from build123d import *

# Parameters (mm, degrees)
SKETCH1_W           = 50
SKETCH1_H           = 50
BOSS_EXTRUDE1_DEPTH = 30
SKETCH2_R           = 2.5
CUT_EXTRUDE1_DEPTH  = 15
CUT_EXTRUDE2_REACH  = 65.443
SKETCH4_R           = 6
SKETCH5_R           = 1.5
CUT_EXTRUDE3_DEPTH  = 10
CUT_EXTRUDE4_START  = -10
SKETCH6_R           = 1.5
CUT_EXTRUDE4_DEPTH  = 10
FILLET1_R           = 4
SKETCH8_R           = 2.5
CUT_EXTRUDE5_DEPTH  = 15


with BuildPart() as part:
    # Sketch1 → Boss-Extrude1 (new body)
    with BuildSketch(Plane(origin=(0, 0, 0), x_dir=(1, 0, 0), z_dir=(0, 1, 0))):
        Rectangle(SKETCH1_W, SKETCH1_H)
    extrude(amount=BOSS_EXTRUDE1_DEPTH)

    # Sketch2 → Cut-Extrude1 (cut)
    with BuildSketch(Plane.XZ):
        with Locations(Location((0, 10, 0), (0, 0, 270))):
            Circle(SKETCH2_R)
        with Locations(Location((0, -10, 0), (0, 0, 270))):
            Circle(SKETCH2_R)
        with Locations(Location((10, 0, 0), (0, 0, 270))):
            Circle(SKETCH2_R)
        with Locations(Location((-10, 0, 0), (0, 0, 270))):
            Circle(SKETCH2_R)
        with Locations(Location((0, 0, 0), (0, 0, 270))):
            Circle(SKETCH2_R)
    extrude(amount=-CUT_EXTRUDE1_DEPTH, mode=Mode.SUBTRACT)

    # Sketch4 → Cut-Extrude2 (cut, up to next)
    with BuildSketch(Plane.ZY.offset(25), mode=Mode.PRIVATE) as cut_extrude2_sk1:
        with Locations((0, 16)):
            Circle(SKETCH4_R)
    cut_extrude2_tool1 = extrude(cut_extrude2_sk1.sketch, amount=-CUT_EXTRUDE2_REACH, mode=Mode.PRIVATE) & part.part
    add(cut_extrude2_tool1.solids().sort_by_distance((-25, 16, 0))[0], mode=Mode.SUBTRACT)

    # Sketch5 → Cut-Extrude3 (cut)
    with BuildSketch(Plane.ZY.offset(25)):
        with Locations((-8, 16)):
            Circle(SKETCH5_R)
        with Locations((8, 16)):
            Circle(SKETCH5_R)
        with Locations((0, 8)):
            Circle(SKETCH5_R)
        with Locations((0, 24)):
            Circle(SKETCH5_R)
    extrude(amount=-CUT_EXTRUDE3_DEPTH, mode=Mode.SUBTRACT)

    # Sketch6 → Cut-Extrude4 (cut)
    with BuildSketch(Plane(origin=(25, 0, 0), x_dir=(0, 0, -1), z_dir=(1, 0, 0)).offset(CUT_EXTRUDE4_START)):
        with Locations(Location((-8, 16, 0), (0, 0, 180))):
            Circle(SKETCH6_R)
        with Locations(Location((8, 16, 0), (0, 0, 180))):
            Circle(SKETCH6_R)
        with Locations(Location((0, 24, 0), (0, 0, 180))):
            Circle(SKETCH6_R)
        with Locations(Location((0, 8, 0), (0, 0, 180))):
            Circle(SKETCH6_R)
    extrude(amount=CUT_EXTRUDE4_DEPTH, mode=Mode.SUBTRACT)

    # Fillet1
    fillet1_edges = [part.edges().sort_by_distance(p)[0] for p in [
        (25, 15, 25),
        (-25, 15, 25),
        (-25, 15, -25),
        (25, 15, -25),
    ]]
    fillet(fillet1_edges, radius=FILLET1_R)

    # Sketch8 → Cut-Extrude5 (cut)
    with BuildSketch(Plane(origin=(0, 30, 0), x_dir=(1, 0, 0), z_dir=(0, 1, 0))):
        with Locations(Location((-16, 16, 0), (0, 0, 270))):
            Circle(SKETCH8_R)
        with Locations(Location((16, 16, 0), (0, 0, 270))):
            Circle(SKETCH8_R)
        with Locations(Location((16, -16, 0), (0, 0, 270))):
            Circle(SKETCH8_R)
        with Locations(Location((-16, -16, 0), (0, 0, 270))):
            Circle(SKETCH8_R)
    extrude(amount=-CUT_EXTRUDE5_DEPTH, mode=Mode.SUBTRACT)


solid = part.part
Can you work these out from the model? Positions are in its coordinate system, mm. A direction names the side the tool comes from. Coordinates: 2 decimals unless noted, no trailing zeros. Order: outer loops, then holes, each group sorted by start corner. A loop starts at its lowest first (then second) coordinate and runs counter-clockwise, first axis right, second up. Notation, with made-up numbers: (-32, 66) -> (-22, 66) arc R28 cw to (-22, 87) -> close; hole circle Ø6 at (-19.5, 49). An arc over 180 degrees is marked (long way). Use one line per item in the form item = value.
Q1. We'd pull the mould along Z, two halves only. Please class faces 6 (the face through (0, 30, 0)), 7 (the face through (-23.859, 15.21, 23.797)), 8 (the face through (-17.5, 22.6, 14)): released by +Z, released by -Z, zero draft, split by the parting line, or undercut.
From the geometry:
face_6 = zero draft
face_7 = released by +Z
face_8 = undercut
Q2. Will these pins go through, and if not, where does the flat tip stop? P1, Ø1.5, axis at y = 16.5, z = 8, coming from the +X side; P2, Ø2.5, axis at y = 8, z = 0, coming from the -X side.
From the geometry:
P1 = 15
P2 = -15
Q3. Imagine slicing it at D-D, the plane x = 5.5. List the corners of the cut face in (y, z) for me.
From the geometry:
outline = (0, -25) -> (30, -25) -> (30, 25) -> (0, 25) -> close; hole circle Ø12 at (16, 0)
Q4. Imagine slicing it at B-B, the plane y = 13. List the corners of the cut face in (x, z) for me.
From the geometry:
outline = (-25, -21) arc R4 ccw to (-21, -25) -> (21, -25) arc R4 ccw to (25, -21) -> (25, -5.2) -> (-25, -5.2) -> close; (-25, 5.2) -> (25, 5.2) -> (25, 21) arc R4 ccw to (21, 25) -> (-21, 25) arc R4 ccw to (-25, 21) -> close; hole circle Ø5 at (0, -10); hole circle Ø5 at (0, 10)
Q5. I need wall thicknesses on L1, parallel to X at y = 22.5, z = 16; L2, parallel to Z at x = 20, y = 8; L3, parallel to X at y = 18, z = -14. Which ranges of each line are inside material? Lowest first, please.
From the geometry:
L1 = -25 to -18.5, -13.5 to 13.5, 18.5 to 25
L2 = -25 to -1.5, 1.5 to 25
L3 = -25 to -17.5, -14.5 to 14.5, 17.5 to 25
Q6. Imagine slicing it at A-A, the plane x = 16. List the corners of the cut face in (y, z) for me, then the cut area to 3 significant figures.
From the geometry:
outline = (0, -25) -> (30, -25) -> (30, -18.5) -> (15, -18.5) -> (15, -13.5) -> (30, -13.5) -> (30, 13.5) -> (15, 13.5) -> (15, 18.5) -> (30, 18.5) -> (30, 25) -> (0, 25) -> close; hole circle Ø3 at (8, 0); hole circle Ø12 at (16, 0); hole circle Ø3 at (16, -8); hole circle Ø3 at (16, 8); hole circle Ø3 at (24, 0)
area = 1,210 mm²
Q7. Which directions (+Z, -Z, +X, -X, +Y, -Y) give clear straight access to the entire face, cutting with the end or side of a thin tool? Please do faces 1 (the face through (-25, 11, 5)), 2 (the face through (19.93, 15.93, 6.5)), 3 (the face through (14.5, 22.6, -18)), 4 (the face through (-20.07, 17.01, 6.89)), 5 (the face through (7.56, 5.2, 0.54)).
From the geometry:
face_1 = +Z, -Z, -X, +Y, -Y
face_2 = +X
face_3 = +Y
face_4 = -X
face_5 = -Y
Q8. Imagine slicing it at C-C, the plane z = -11.5. List the corners of the cut face in (x, y) for me.
From the geometry:
outline = (-25, 0) -> (-2, 0) -> (-2, 15) -> (2, 15) -> (2, 0) -> (25, 0) -> (25, 30) -> (-25, 30) -> close
